```python
from build123d import *

# Parameters (mm, degrees)
SKETCH1_W            = 115
SKETCH1_H            = 55
BOSS_EXTRUDE1_DEPTH  = 30
SKETCH2_W            = 88
SKETCH2_H            = 22
CUT_EXTRUDE1_DEPTH   = 86.036756758
SHELL1_T             = 5
M4_CLEARANCE_HOLE1_D = 4.8
CHAMFER1_SIZE        = 2
FILLET1_R            = 6
FILLET2_R            = 6


with BuildPart() as part:
    # Sketch1 → Boss-Extrude1 (new body)
    with BuildSketch(Plane.XY):
        Rectangle(SKETCH1_W, SKETCH1_H)
    extrude(amount=BOSS_EXTRUDE1_DEPTH)

    # Sketch2 → Cut-Extrude1 (cut, through all)
    with BuildSketch(Plane(origin=(0, 27.5, 0), x_dir=(1, 0, 0), z_dir=(0, 1, 0))):
        with Locations((9, -19)):
            Rectangle(SKETCH2_W, SKETCH2_H)
    extrude(amount=-CUT_EXTRUDE1_DEPTH, mode=Mode.SUBTRACT)

    # Shell1
    shell1_openings = [part.faces().sort_by_distance(p)[0] for p in [
        (0, -27.5, 1.188486432),
        (55.25, 0, 30),
        (53, 0, 19),
        (9, 0, 8),
        (-35, 0, 19),
        (-46.25, 0, 30),
    ]]
    offset(amount=SHELL1_T, openings=shell1_openings, kind=Kind.INTERSECTION)

    # M4 Clearance Hole1 (through all)
    with Locations(Plane.ZY.offset(62.5)):
        with Locations((17.5, -14.5)):
            Hole(M4_CLEARANCE_HOLE1_D / 2)

    # Chamfer1
    chamfer1_edges = [part.edges().sort_by_distance(p)[0] for p in [
        (-35, 30, 30),
        (53, 30, 30),
        (0, -27.5, -5),
        (-62.5, 2.5, -5),
        (0, 32.5, -5),
        (62.5, 2.5, -5),
        (-62.5, 32.5, 12.5),
        (62.5, 32.5, 12.5),
    ]]
    chamfer(chamfer1_edges, length=CHAMFER1_SIZE)

    # Fillet1
    fillet1_edges = [part.edges().sort_by_distance(p)[0] for p in [
        (-35, 30, 8),
        (53, 30, 8),
    ]]
    fillet(fillet1_edges, radius=FILLET1_R)

    # Fillet2
    fillet2_edges = [part.edges().sort_by_distance(p)[0] for p in [
        (60, -27.5, 30),
        (-60, -27.5, 30),
    ]]
    fillet(fillet2_edges, radius=FILLET2_R)


solid = part.part
```
Could you check a few things on this model? Use its own coordinates, in mm. A direction names the side the tool comes from. Coordinates: 2 decimals unless noted, no trailing zeros. Write each loop counter-clockwise with the first axis right and the second up, starting at its lowest first coordinate (ties: lowest second). Pieces come first, ordered by that corner, then holes. Notation, with made-up numbers: (2, 82.25) - (10, 82.25) arc R20 ccw to (10, 120.25) - close; hole circle Ø6 at (65.25, 59.5). An arc over 180 degrees is marked (long way). Use a Markdown table: item, result.
Q1. Imagine slicing it at C-C (x = -47.5). List the corners of the cut face in (y, z) for me, and give its area (3 significant figures).
Geometry check:
| item | result |
|---|---|
| outline | (-27.5, -3) - (-25.5, -5) - (30.5, -5) - (32.5, -3) - (32.5, 30) - (27.5, 30) - (27.5, 0) - (-27.5, 0) - close |
| area | 446 mm2 |
Q2. Which directions (+Z, -Z, +X, -X, +Y, -Y) give clear straight access to the entire face, cutting with the end or side of a thin tool? Please do faces 1 (the flat face through (-57.5, 0, 15)), 2 (the flat face through (53, 30, 21)), 3 (the cylindrical face through (60.04, -12.12, 17.81)).
Geometry check:
| item | result |
|---|---|
| face 1 | +Z, -Y |
| face 2 | +Z, +Y, -Y |
| face 3 | +X, -X |
Q3. Imagine slicing it at D-D (z = 2). List the corners of the cut face in (x, y) for me, and give its area (3 significant figures).
Geometry check:
| item | result |
|---|---|
| outline | (-62.5, -27.5) - (-57.5, -27.5) - (-57.5, 27.5) - (57.5, 27.5) - (57.5, -27.5) - (62.5, -27.5) - (62.5, 30.5) - (60.5, 32.5) - (-60.5, 32.5) - (-62.5, 30.5) - close |
| area | 1,170 mm2 |
Q4. Please list where these lines run through material, in increasing order: L1, parallel to X at y = 19.5, z = 7.5; L2, parallel to Z at x = -27.5, y = 8.5; L3, parallel to Y at x = -42.5, z = 14.
Geometry check:
| item | result |
|---|---|
| L1 | x = -62.5 to -57.5, 57.5 to 62.5 |
| L2 | z = -5 to 0 |
| L3 | y = 27.5 to 32.5 |
Q5. I'm going to push flat-ended pins straight in: pin 1 Ø5.5 at (y, z) = (-14.5, 17.5) entering from +X; pin 2 Ø8 at (x, y) = (-26, -6) entering from +Z; pin 3 Ø4 at (x, y) = (21.5, 30) entering from +Z. Where does each tip first touch, or does it pass through?
Geometry check:
| item | result |
|---|---|
| pin 1 | stops at x = 62.5 |
| pin 2 | stops at z = 0 |
| pin 3 | stops at z = 8 |
Q6. Imagine slicing it at B-B (y = -14.5). List the corners of the cut face in (x, z) for me.
Geometry check:
| item | result |
|---|---|
| outline | (-62.5, -3) - (-60.5, -5) - (60.5, -5) - (62.5, -3) - (62.5, 15.1) - (57.5, 15.1) - (57.5, 0) - (-57.5, 0) - (-57.5, 15.1) - (-62.5, 15.1) - close; (-62.5, 19.9) - (-57.5, 19.9) - (-57.5, 30) - (-62.5, 30) - close; (57.5, 19.9) - (62.5, 19.9) - (62.5, 30) - (57.5, 30) - close |
Q7. Imagine slicing it at A-A (z = 17.5). List the corners of the cut face in (x, y) for me.
Geometry check:
| item | result |
|---|---|
| outline | (-62.5, -27.5) - (-57.5, -27.5) - (-57.5, -16.9) - (-62.5, -16.9) - close; (-62.5, -12.1) - (-57.5, -12.1) - (-57.5, 27.5) - (-35, 27.5) - (-35, 32.5) - (-60.5, 32.5) - (-62.5, 30.5) - close; (53, 27.5) - (57.5, 27.5) - (57.5, -12.1) - (62.5, -12.1) - (62.5, 30.5) - (60.5, 32.5) - (53, 32.5) - close; (57.5, -27.5) - (62.5, -27.5) - (62.5, -16.9) - (57.5, -16.9) - close |
Q8. Thinking about a two-plate mould opening in X: for faces 4 (the flat face through (-62.5, 1, 13)), 5 (the flat face through (-35, 30, 21)), 6 (the cylindrical face through (-59.965, -25.696, 28.289)), which applies, +X half, -X half, draft (parallel to the pull), parting line (faces both ways), or undercut?
Geometry check:
| item | result |
|---|---|
| face 4 | -X half |
| face 5 | undercut |
| face 6 | draft |
